from build123d import *

# Parameters (mm, degrees)
CROQUIS1_W              = 30
CROQUIS1_H              = 80.8
SALIENTE_EXTRUIR1_DEPTH = 4
CROQUIS3_R              = 2
CORTAR_EXTRUIR2_DEPTH   = 5
CROQUIS8_R              = 2.55
CORTAR_EXTRUIR3_DEPTH   = 5
CROQUIS10_R             = 3.05
CORTAR_EXTRUIR4_DEPTH   = 2
CROQUIS11_R             = 1.575
CORTAR_EXTRUIR5_DEPTH   = 3
CHAFL_N1_SIZE           = 3


with BuildPart() as part:
    # Croquis1 → Saliente-Extruir1 (new body)
    with BuildSketch(Plane(origin=(0, 0, 0), x_dir=(0, 0, -1), z_dir=(1, 0, 0))):
        Rectangle(CROQUIS1_W, CROQUIS1_H)
    extrude(amount=SALIENTE_EXTRUIR1_DEPTH)

    # Croquis3 → Cortar-Extruir2 (cut, through all)
    with BuildSketch(Plane(origin=(4, 0, 0), x_dir=(0, 0, -1), z_dir=(1, 0, 0))):
        with Locations((-10, -12.5)):
            Circle(CROQUIS3_R)
        with Locations((10, -12.5)):
            Circle(CROQUIS3_R)
        with Locations((-10, -32.5)):
            Circle(CROQUIS3_R)
        with Locations((10, -32.5)):
            Circle(CROQUIS3_R)
    extrude(amount=-CORTAR_EXTRUIR2_DEPTH, mode=Mode.SUBTRACT)

    # Croquis8 → Cortar-Extruir3 (cut, through all)
    with BuildSketch(Plane.ZY):
        with Locations((0, 23.15)):
            Circle(CROQUIS8_R)
    extrude(amount=-CORTAR_EXTRUIR3_DEPTH, mode=Mode.SUBTRACT)

    # Croquis10 → Cortar-Extruir4 (cut)
    with BuildSketch(Plane.ZY.offset(-4)):
        with Locations((-10.4, 34.85)):
            Circle(CROQUIS10_R)
        with Locations((10.4, 34.85)):
            Circle(CROQUIS10_R)
        with Locations((10.4, 2.5)):
            Circle(CROQUIS10_R)
        with Locations((-10.4, 2.5)):
            Circle(CROQUIS10_R)
    extrude(amount=CORTAR_EXTRUIR4_DEPTH, mode=Mode.SUBTRACT)

    # Croquis11 → Cortar-Extruir5 (cut, through all)
    with BuildSketch(Plane(origin=(2, 0, 0), x_dir=(0, 0, -1), z_dir=(1, 0, 0))):
        with Locations((-10.4, 34.85)):
            Circle(CROQUIS11_R)
        with Locations((10.4, 34.85)):
            Circle(CROQUIS11_R)
        with Locations((10.4, 2.5)):
            Circle(CROQUIS11_R)
        with Locations((-10.4, 2.5)):
            Circle(CROQUIS11_R)
    extrude(amount=-CORTAR_EXTRUIR5_DEPTH, mode=Mode.SUBTRACT)

    # Chaflán1
    chafl_n1_edges = [part.edges().sort_by_distance(p)[0] for p in [
        (2, 40.4, 15),
        (2, 40.4, -15),
    ]]
    chamfer(chafl_n1_edges, length=CHAFL_N1_SIZE)


solid = part.part
The listing builds one solid part. Answer for the finished solid, in the listing's coordinates (mm). A direction names the side the tool comes from. Round coordinates to 2 decimals unless told otherwise and drop trailing zeros. Order: outer loops, then holes, each group sorted by start corner. A loop starts at its lowest first (then second) coordinate and runs counter-clockwise, first axis right, second up. Notation, with made-up numbers: (24.5, 81) -> (56.5, 81) arc R23 cw to (56.5, 89) -> close; hole circle Ø5 at (-22, 79). An arc over 180 degrees is marked (long way). Write each question's results on one line, items separated by ' | '. Start each with the question number.
Q1. The mould has two halves that part along Z. Classify faces 1 (the cylindrical face through (3.014, 2.634, -13.447)), 2 (the flat face through (2, -40.4, 0)), 3 (the flat face through (2, 38.9, 13.5)): pulls with the +Z half, pulls with the -Z half, needs draft (parallel to the pull), parting line crosses it, or undercut.
Q2. Find section B-B (x = 2.6). Give the number of separate pieces and of enclosed holes in the cut face, then the cut area to 3 significant figures.
Q3. Which of the six approach directions +Z, -Z, +X, -X, +Y, -Y give full straight-line access (tool end or side, diameter ignored) to faces 4 (the cylindrical face through (1.01, 36.41, 10.61)), 5 (the cylindrical face through (3.014, 37.874, -10.797))?
Q4. Find section A-A (y = 2.5). Determine the outline of the cut face in (x, z) (3 decimals).
Q5. Find section D-D (z = -10.4). Determine the outline of the cut face in (x, y) (3 decimals).
Q6. Each of these flat-tipped pins is pushed along its axis until it touches: pin 1 (5 mm diameter, centred on y = 1.5, z = -10, fed in from +X); pin 2 (3 mm diameter, centred on y = 2.5, z = 10.4, fed in from -X); pin 3 (5 mm diameter, centred on y = 34.85, z = -10.4, fed in from +X). Where does it stop, or does it pass through?
Q7. Straight lines are drawn through the part: probe 1 along Z at (x, y) = (1.55, -31.5); probe 2 along Y at (x, z) = (1.85, -10); probe 3 along Y at (x, z) = (2.4, 10). For each, find the intervals that lie inside material, in ascending order. Write a range as from..to.
Q8. Find section C-C (y = 23.15). Determine the outline of the cut face in (x, z).
Worked answers:
1) face 1: undercut | face 2: needs draft | face 3: pulls with the +Z half
2) separate pieces: 1 | enclosed holes: 9 | area: 2,230 mm2
3) face 4: +X, -X | face 5: +X
4) outline: (0, -15) -> (4, -15) -> (4, -13.45) -> (2, -13.45) -> (2, -11.975) -> (0, -11.975) -> close; (0, -8.825) -> (2, -8.825) -> (2, -7.35) -> (4, -7.35) -> (4, 7.35) -> (2, 7.35) -> (2, 8.825) -> (0, 8.825) -> close; (0, 11.975) -> (2, 11.975) -> (2, 13.45) -> (4, 13.45) -> (4, 15) -> (0, 15) -> close
5) outline: (0, -40.4) -> (4, -40.4) -> (4, -34.46) -> (0, -34.46) -> close; (0, -30.54) -> (4, -30.54) -> (4, -14.46) -> (0, -14.46) -> close; (0, -10.54) -> (4, -10.54) -> (4, -0.55) -> (2, -0.55) -> (2, 0.925) -> (0, 0.925) -> close; (0, 4.075) -> (2, 4.075) -> (2, 5.55) -> (4, 5.55) -> (4, 31.8) -> (2, 31.8) -> (2, 33.275) -> (0, 33.275) -> close; (0, 36.425) -> (2, 36.425) -> (2, 37.9) -> (4, 37.9) -> (4, 40.4) -> (0, 40.4) -> close
6) pin 1: stops at x = 4 | pin 2: passes through | pin 3: stops at x = 2
7) probe 1: z = -15..-11.73, -8.27..8.27, 11.73..15 | probe 2: y = -40.4..-34.5, -30.5..-14.5, -10.5..0.98, 4.02..33.33, 36.37..40.4 | probe 3: y = -40.4..-34.5, -30.5..-14.5, -10.5..-0.52, 5.52..31.83, 37.87..40.4
8) outline: (0, -15) -> (4, -15) -> (4, -2.55) -> (0, -2.55) -> close; (0, 2.55) -> (4, 2.55) -> (4, 15) -> (0, 15) -> close
